Read the model definition and answer for the solid it produces. Units are mm, in the model's axes. Coordinates: 2 decimals unless noted, no trailing zeros. Order: outer loops, then holes, each group sorted by start corner. A loop starts at its lowest first (then second) coordinate and runs counter-clockwise, first axis right, second up. Notation, with made-up numbers: M 54.25,22 L 99.25,22 A25 ccw 99.25,42 Z; hole C -7,60.5 d4. An arc over 180 degrees is marked long. Put each result on its own line as item: value.
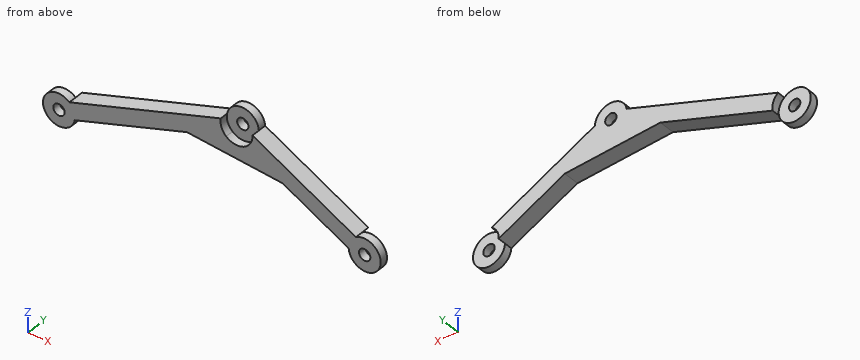
from build123d import *

# Parameters (mm, degrees)
SKETCH2_R           = 2.2479
BOSS_EXTRUDE2_DEPTH = 6.35
CUT_EXTRUDE1_START  = -3.175
SKETCH3_R           = 6.35
CUT_EXTRUDE1_DEPTH  = 3.175
SKETCH4_R           = 6.35
CUT_EXTRUDE2_DEPTH  = 3.175
BOSS_EXTRUDE3_START = -6.35
BOSS_EXTRUDE3_DEPTH = 6.35


with BuildPart() as part:
    # Sketch2 → Boss-Extrude2 (new body)
    with BuildSketch(Plane(origin=(0, 0, 0), x_dir=(1, 0, 0), z_dir=(0, 1, 0))):
        with BuildLine():
            Line((76.696592015, -25.780461907), (117.659214316, -5.299150756))
            ThreePointArc((117.659214316, -5.299150756), (126.837612663, 2.839806331), (114.819407985, 0.380461907))
            Line((114.819407985, 0.380461907), (73.856785684, -20.100849244))
            ThreePointArc((73.856785684, -20.100849244), (69.986110983, -19.060899231), (66.263588885, -20.546310927))
            Line((66.263588885, -20.546310927), (6.250623597, 1.119019502))
            ThreePointArc((6.250623597, 1.119019502), (-5.972708576, 2.156212482), (4.094411115, -4.853689073))
            Line((4.094411115, -4.853689073), (64.107376403, -26.519019502))
            ThreePointArc((64.107376403, -26.519019502), (70.729889017, -31.739100769), (76.696592015, -25.780461907))
        make_face()
        with Locations(Location((70.358, -25.4, 0), (0, 0, 270))):
            Circle(SKETCH2_R, mode=Mode.SUBTRACT)
        with Locations(Location((0, 0, 0), (0, 0, 270))):
            Circle(SKETCH2_R, mode=Mode.SUBTRACT)
        with Locations(Location((121.158, 0, 0), (0, 0, 270))):
            Circle(SKETCH2_R, mode=Mode.SUBTRACT)
    extrude(amount=BOSS_EXTRUDE2_DEPTH)

    # Sketch3 → Cut-Extrude1 (cut)
    with BuildSketch(Plane(origin=(0, 6.35, 0), x_dir=(1, 0, 0), z_dir=(0, 1, 0)).offset(CUT_EXTRUDE1_START)):
        Circle(SKETCH3_R)
        with Locations((121.158, 0)):
            Circle(SKETCH3_R)
    extrude(amount=CUT_EXTRUDE1_DEPTH, mode=Mode.SUBTRACT)

    # Sketch4 → Cut-Extrude2 (cut)
    with BuildSketch(Plane.XZ):
        with Locations((70.358, 25.4)):
            Circle(SKETCH4_R)
    extrude(amount=-CUT_EXTRUDE2_DEPTH, mode=Mode.SUBTRACT)

    # Sketch5 → Boss-Extrude3 (add)
    with BuildSketch(Plane(origin=(0, 6.35, 0), x_dir=(1, 0, 0), z_dir=(0, 1, 0)).offset(BOSS_EXTRUDE3_START)):
        with BuildLine():
            Line((88.623778607, -12.717352782), (73.856785684, -20.100849244))
            ThreePointArc((73.856785684, -20.100849244), (69.986110983, -19.060899231), (66.263588885, -20.546310927))
            Line((66.263588885, -20.546310927), (50.734546588, -14.940158473))
            Line((50.734546588, -14.940158473), (88.623778607, -12.717352782))
        make_face()
    extrude(amount=BOSS_EXTRUDE3_DEPTH)


solid = part.part
Q1. Find section C-C on x = 38. Write down the section's boundary in (y, z).
Answers below:
outline: M 0,10.34 L 6.35,10.34 L 6.35,17.09 L 0,17.09 Z
Q2. Consider line 1 along Z through (x, y) = (0, 2.45); line 2 along X through (y, z) = (1.75, -4.5); line 3 along Z through (x, y) = (32, 0.75). Determine where each line is inside the solid, lowest interval first.
Answers below:
line 1: z = -6.35 to -2.25, 2.25 to 6.35
line 2: x = -4.48 to 4.48, 116.68 to 125.64
line 3: z = 8.18 to 14.93
Q3. Given pin 1 (1.5 mm diameter, centred on x = 48.5, y = 4, fed in from +Z); pin 2 (6.5 mm diameter, centred on x = 124, z = 2, fed in from +Y) (3 decimals); pin 3 (2 mm diameter, centred on x = 62, y = 1, fed in from +Z), each flat-ended and moving along its own axis, determine where each tip first touches the part or whether it passes through.
Answers below:
pin 1: stops at z = 21.16
pin 2: stops at y = 3.175
pin 3: stops at z = 26.12
Q4. Find section A-A on x = 0. Write down the section's boundary in (y, z) (3 decimals).
Answers below:
outline: M 0,-6.35 L 3.175,-6.35 L 3.175,-2.248 L 0,-2.248 Z; M 0,2.248 L 3.175,2.248 L 3.175,6.35 L 0,6.35 Z
Q5. Find section B-B on y = 1. Write down the section's boundary in (x, z), plus the area to 3 significant figures.
Answers below:
outline: M 4.09,4.85 A6.35 ccw long 6.25,-1.12 L 50.73,14.94 L 88.62,12.72 L 114.82,-0.38 A6.35 ccw long 117.66,5.3 L 76.7,25.78 A6.35 cw long 64.11,26.52 Z; hole C 0,0 d4.5; hole C 121.16,0 d4.5
area: 1,040 mm^2
